The listing builds one solid part. Answer for the finished solid, in the listing's coordinates (mm). Face numbers are marked on the shaded views. A direction names the side the tool comes from. Give positions to 0.01 mm unless a question says otherwise; leave off trailing zeros. Loops run counter-clockwise (first coordinate to the right, second up) from the corner with the lowest first, then second, coordinate; pieces in that order, holes last. Notation, with made-up numbers: (24, -24.75) - (66, -24.75) arc R31 cw to (66, 14.25) - close; hole circle Ø1 at (5.5, -31). An arc over 180 degrees is marked (long way). One line per item, written item: value. Start each with the question number.
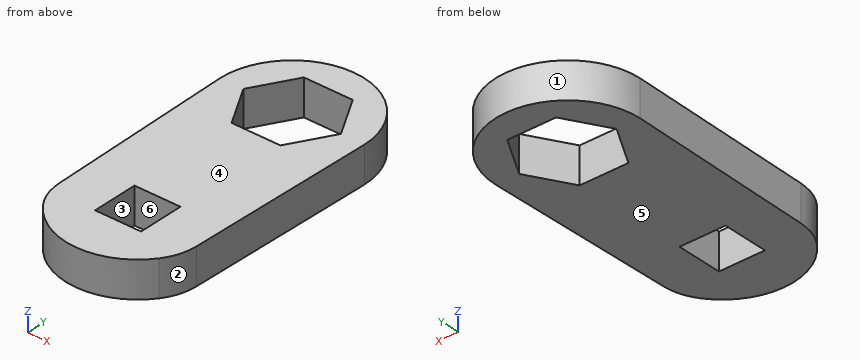
from build123d import *

# Parameters (mm, degrees)
SKETCH_W  = 12.75
SKETCH_H  = 12.75
PAD_DEPTH = 10
FILLET_R  = 15


with BuildPart() as part:
    # Sketch → Pad (new body)
    with BuildSketch(Plane.XY):
        with BuildLine():
            ThreePointArc((20, 0), (0, 20), (-20, 0))
            Line((-20, 0), (-18.956776, -56.375))
            ThreePointArc((-18.956776, -56.375), (0, -70), (18.956776, -56.375))
            Line((18.956776, -56.375), (20, 0))
        make_face()
        Polygon((-13.525, 0), (-6.7625, -11.712994), (6.7625, -11.712994), (13.525, 0), (6.7625, 11.712994), (-6.7625, 11.712994), align=None, mode=Mode.SUBTRACT)
        with Locations((0, -50)):
            Rectangle(SKETCH_W, SKETCH_H, mode=Mode.SUBTRACT)
    extrude(amount=PAD_DEPTH)

    # Fillet
    fillet_edges = [part.edges().sort_by_distance(p)[0] for p in [
        (-20, 0, 5),
        (-18.956776, -56.375, 5),
        (18.956776, -56.375, 5),
        (20, 0, 5),
    ]]
    fillet(fillet_edges, radius=FILLET_R)


solid = part.part
1. A cutting plane is placed at D-D (x = -4.5). Determine the outline of the cut face in (y, z) (3 decimals).
2. A cutting plane is placed at B-B (z = 3). Determine the outline of the cut face in (x, y) (1 decimal), plus the area to 3 significant figures.
3. For the marked faces 5 and 6, determine the directions among +Z, -Z, +X, -X, +Y, -Y from which every point of the face is accessible in a straight line to the end or side of a thin tool.
4. Find the intervals of material crossed by L1, parallel to Y at x = -4, z = 3.25 (3 decimals); L2, parallel to Y at x = -2, z = 7.75 (3 decimals); L3, parallel to X at y = -50, z = 9.25 (3 decimals), in increasing order. Write a range as [from, to].
5. A cutting plane is placed at A-A (x = 0). Determine the outline of the cut face in (y, z) (3 decimals).
6. Flat-ended cylindrical pins translate along their axes: pin 1 (12 mm diameter, centred on x = -4.5, y = 1.5, fed in from +Z); pin 2 (5 mm diameter, centred on y = -33.5, z = 3, fed in from -X); pin 3 (3 mm diameter, centred on y = -53, z = 3, fed in from +X); pin 4 (3 mm diameter, centred on x = 1, z = 5.5, fed in from -Y). Find the tip coordinate at first contact, or state that the pin passes through.
7. A cutting plane is placed at C-C (y = 9). Determine the outline of the cut face in (x, z).
8. Determine the mould class of the marked faces 1, 2, 3 and 4 for opening direction X: released by +X, released by -X, zero draft, split by the parting line, or undercut.
Results below:
1. outline: (-69.487, 0) - (-56.375, 0) - (-56.375, 10) - (-69.487, 10) - close; (-43.625, 0) - (-11.713, 0) - (-11.713, 10) - (-43.625, 10) - close; (11.713, 0) - (19.487, 0) - (19.487, 10) - (11.713, 10) - close
2. outline: (-20, 0) - (-19, -53.3) arc R15 ccw to (-16.1, -61.9) arc R20 ccw to (16.1, -61.9) arc R15 ccw to (19, -53.3) - (20, 0) arc R20 ccw to start; hole (-13.5, 0) - (-6.8, -11.7) - (6.8, -11.7) - (13.5, 0) - (6.8, 11.7) - (-6.8, 11.7) - close; hole (-6.4, -56.4) - (6.4, -56.4) - (6.4, -43.6) - (-6.4, -43.6) - close
2. area: 2,560 mm^2
3. face 5: -Z, +X, -X, +Y, -Y
3. face 6: +Z, -Z
4. L1: y = [-69.596, -56.375], [-43.625, -11.713], [11.713, 19.596]
4. L2: y = [-69.9, -56.375], [-43.625, -11.713], [11.713, 19.9]
4. L3: x = [-19.075, -6.375], [6.375, 19.075]
5. outline: (-70, 0) - (-56.375, 0) - (-56.375, 10) - (-70, 10) - close; (-43.625, 0) - (-11.713, 0) - (-11.713, 10) - (-43.625, 10) - close; (11.713, 0) - (20, 0) - (20, 10) - (11.713, 10) - close
6. pin 1: passes through
6. pin 2: stops at x = -19.43
6. pin 3: stops at x = 19.05
6. pin 4: stops at y = -70
7. outline: (-17.86, 0) - (-8.33, 0) - (-8.33, 10) - (-17.86, 10) - close; (8.33, 0) - (17.86, 0) - (17.86, 10) - (8.33, 10) - close
8. face 1: split by the parting line
8. face 2: released by +X
8. face 3: undercut
8. face 4: zero draft
